Read the model definition and answer for the solid it produces. Units are mm, in the model's axes. A direction names the side the tool comes from. Coordinates: 2 decimals unless noted, no trailing zeros. Loops run counter-clockwise (first coordinate to the right, second up) from the corner with the lowest first, then second, coordinate; pieces in that order, holes last. Notation, with made-up numbers: (-1.75, 18) -> (38.25, 18) arc R24 cw to (38.25, 46) -> close; hole circle Ø8 at (-37, 55). An arc over 180 degrees is marked (long way). One line per question, with ' | ' between items. Start each with the question number.
```python
from build123d import *

# Parameters (mm, degrees)
SKETCH1_R           = 2.4892
BOSS_EXTRUDE1_DEPTH = 3.175
FILLET1_R           = 6.35
LPATTERN1_START     = -3.175
LPATTERN1_OUTLINE_R = 2.4892
LPATTERN1_DEPTH     = 6.35
SKETCH2_R           = 2.4892
SKETCH2_W           = 190.5
SKETCH2_H           = 254
CUT_EXTRUDE1_DEPTH  = 353.596579854
FILLET2_R           = 8.255


# Read off the part's stored shape, not the designer's step: LPattern1
with BuildPart() as part:
    # Sketch1 → Boss-Extrude1 (new, symmetric)
    with BuildSketch(Plane(origin=(0, 0, 0), x_dir=(1, 0, 0), z_dir=(0, 1, 0))):
        Polygon((0, 50.8), (0, 0), (215.9, 0), (215.9, 50.8), (244.475, 50.8), (244.475, 203.2), (215.9, 203.2), (215.9, 254), (0, 254), (0, 203.2), (-28.575, 203.2), (-28.575, 50.8), align=None)
        Polygon((12.7, 190.5), (12.7, 219.075), (190.5, 219.075), (190.5, 190.5), (212.725, 190.5), (212.725, 63.5), (190.5, 63.5), (190.5, 34.925), (12.7, 34.925), (12.7, 63.5), (-9.525, 63.5), (-9.525, 190.5), align=None, mode=Mode.SUBTRACT)
        with Locations(Location((209.55, 12.7, 0), (0, 0, 270))):
            Circle(SKETCH1_R, mode=Mode.SUBTRACT)
        with BuildLine():
            Line((227.0125, 142.875), (227.0125, 111.125))
            ThreePointArc((227.0125, 111.125), (222.25, 106.3625), (217.4875, 111.125))
            Line((217.4875, 111.125), (217.4875, 142.875))
            ThreePointArc((217.4875, 142.875), (222.25, 147.6375), (227.0125, 142.875))
        make_face(mode=Mode.SUBTRACT)
        with BuildLine():
            ThreePointArc((-14.2875, 111.125), (-19.05, 106.3625), (-23.8125, 111.125))
            Line((-23.8125, 111.125), (-23.8125, 142.875))
            ThreePointArc((-23.8125, 142.875), (-19.05, 147.6375), (-14.2875, 142.875))
            Line((-14.2875, 142.875), (-14.2875, 111.125))
        make_face(mode=Mode.SUBTRACT)
        with Locations(Location((209.55, 241.3, 0), (0, 0, 270))):
            Circle(SKETCH1_R, mode=Mode.SUBTRACT)
    extrude(amount=BOSS_EXTRUDE1_DEPTH, both=True)

    # Fillet1
    fillet1_edges = [part.edges().sort_by_distance(p)[0] for p in [
        (0, 0, 0),
        (0, 0, -50.8),
        (-28.575, 0, -50.8),
        (-28.575, 0, -203.2),
        (0, 0, -203.2),
        (0, 0, -254),
        (215.9, 0, -254),
        (215.9, 0, -203.2),
        (244.475, 0, -203.2),
        (244.475, 0, -50.8),
        (215.9, 0, -50.8),
        (215.9, 0, 0),
        (212.725, 0, -190.5),
        (190.5, 0, -190.5),
        (190.5, 0, -219.075),
        (12.7, 0, -219.075),
        (12.7, 0, -190.5),
        (-9.525, 0, -190.5),
        (-9.525, 0, -63.5),
        (12.7, 0, -63.5),
        (12.7, 0, -34.925),
        (190.5, 0, -34.925),
        (190.5, 0, -63.5),
        (212.725, 0, -63.5),
    ]]
    fillet(fillet1_edges, radius=FILLET1_R)

    # LPattern1 outline → LPattern1 (cut)
    with BuildSketch(Plane(origin=(0, 0, 0), x_dir=(1, 0, 0), z_dir=(0, 1, 0)).offset(LPATTERN1_START)):
        with Locations((31.75, 12.7)):
            Circle(LPATTERN1_OUTLINE_R)
        with Locations((31.75, 241.3)):
            Circle(LPATTERN1_OUTLINE_R)
        with Locations((57.15, 12.7)):
            Circle(LPATTERN1_OUTLINE_R)
        with Locations((57.15, 241.3)):
            Circle(LPATTERN1_OUTLINE_R)
        with Locations((82.55, 12.7)):
            Circle(LPATTERN1_OUTLINE_R)
        with Locations((82.55, 241.3)):
            Circle(LPATTERN1_OUTLINE_R)
        with Locations((107.95, 12.7)):
            Circle(LPATTERN1_OUTLINE_R)
        with Locations((107.95, 241.3)):
            Circle(LPATTERN1_OUTLINE_R)
        with Locations((133.35, 12.7)):
            Circle(LPATTERN1_OUTLINE_R)
        with Locations((133.35, 241.3)):
            Circle(LPATTERN1_OUTLINE_R)
        with Locations((158.75, 12.7)):
            Circle(LPATTERN1_OUTLINE_R)
        with Locations((158.75, 241.3)):
            Circle(LPATTERN1_OUTLINE_R)
        with Locations((184.15, 12.7)):
            Circle(LPATTERN1_OUTLINE_R)
        with Locations((184.15, 241.3)):
            Circle(LPATTERN1_OUTLINE_R)
    extrude(amount=LPATTERN1_DEPTH, mode=Mode.SUBTRACT)

    # Sketch2 → Cut-Extrude1 (cut, through all)
    with BuildSketch(Plane(origin=(0, 3.175, 0), x_dir=(1, 0, 0), z_dir=(0, 1, 0))):
        with Locations(Location((234.95, 190.5, 0), (0, 0, 270))):
            Circle(SKETCH2_R)
        with Locations(Location((234.95, 63.5, 0), (0, 0, 270))):
            Circle(SKETCH2_R)
        with Locations((66.675, 127)):
            Rectangle(SKETCH2_W, SKETCH2_H)
    extrude(amount=-CUT_EXTRUDE1_DEPTH, mode=Mode.SUBTRACT)

    # Fillet2
    fillet2_edges = [part.edges().sort_by_distance(p)[0] for p in [
        (161.925, 0, -34.925),
        (161.925, 0, -219.075),
        (161.925, 0, -254),
        (161.925, 0, 0),
    ]]
    fillet(fillet2_edges, radius=FILLET2_R)


solid = part.part
```
(1) Section D-D on y = -0.75 is taken. Give the number of separate pieces and of enclosed holes in the cut face, plus the area to 3 significant figures.
(2) A tool of negligible diameter and unlimited length cuts with its end or side. For faces 1 (the flat face through (230, 3.175, -129)), 2 (the flat face through (215.9, 0, -228)), 3 (the cylindrical face through (222.355, -0.044, -106.364)), 4 (the cylindrical face through (188.689, 0.044, -217.165)), 5 (the cylindrical face through (164.28, -0.04, -2.48)), from which of +Z, -Z, +X, -X, +Y, -Y can it reach the whole face along a straight path? Write none if from no direction.
(3) Each of these flat-tipped pins is pushed along its axis until it touches: pin 1 Ø3 at (y, z) = (0.5, -232.5) entering from +X; pin 2 Ø1 at (y, z) = (0, -49) entering from -X; pin 3 Ø4.5 at (x, z) = (234.95, -63.5) entering from -Y; pin 4 Ø1 at (y, z) = (2, -51) entering from +X. Where does it stop, or does it pass through?
(4) Find the intervals of material crossed by probe 1 along Z at (x, y) = (184.15, 1) (3 decimals); probe 2 along Z at (x, y) = (234.95, -2); probe 3 along Z at (x, y) = (234.5, -2), in increasing order. Write a range as from..to.
(5) Determine the mould class of faces 6 (the flat face through (215.9, 0, -25)), 7 (the flat face through (230, 0, -50.8)), 8 (the flat face through (177, 0, -34.925)), 9 (the cylindrical face through (217.71, 0.04, -205.11)) for opening direction Z: +Z half, -Z half, draft (parallel to the pull), parting line (faces both ways), or undercut.
(6) Section C-C on z = -241.3 is taken. Write down the section's boundary in (x, y) (3 decimals).
(7) Section A-A on z = -119 is taken. Write down the section's boundary in (x, y) (1 decimal).
(8) Section B-B on x = 234.95 is taken. Write down the section's boundary in (y, z) (3 decimals), plus the area to 3 significant figures.
Working result:
1) separate pieces: 1 | enclosed holes: 7 | area: 9,430 mm2
2) face 1: +Z, -Z, +X, -X, +Y | face 2: -Z, +X, +Y, -Y | face 3: +Y, -Y | face 4: -X, +Y, -Y | face 5: +Z, -X, +Y, -Y
3) pin 1: stops at x = 215.9 | pin 2: stops at x = 190.5 | pin 3: passes through | pin 4: stops at x = 241.02
4) probe 1: z = -254..-243.789, -238.811..-219.075, -34.925..-15.189, -10.211..0 | probe 2: z = -203.2..-192.99, -188.01..-65.99, -61.01..-50.8 | probe 3: z = -203.2..-192.95, -188.05..-65.95, -61.05..-50.8
5) face 6: draft | face 7: +Z half | face 8: undercut | face 9: -Z half
6) outline: (161.925, -3.175) -> (181.661, -3.175) -> (181.661, 3.175) -> (161.925, 3.175) -> close; (186.639, -3.175) -> (207.061, -3.175) -> (207.061, 3.175) -> (186.639, 3.175) -> close; (212.039, -3.175) -> (215.9, -3.175) -> (215.9, 3.175) -> (212.039, 3.175) -> close
7) outline: (212.7, -3.2) -> (217.5, -3.2) -> (217.5, 3.2) -> (212.7, 3.2) -> close; (227, -3.2) -> (244.5, -3.2) -> (244.5, 3.2) -> (227, 3.2) -> close
8) outline: (-3.175, -203.2) -> (3.175, -203.2) -> (3.175, -192.989) -> (-3.175, -192.989) -> close; (-3.175, -188.011) -> (3.175, -188.011) -> (3.175, -65.989) -> (-3.175, -65.989) -> close; (-3.175, -61.011) -> (3.175, -61.011) -> (3.175, -50.8) -> (-3.175, -50.8) -> close | area: 905 mm2
